Part print with two shaded views. Sizes in mm from the minimum x, y, z corner. Coordinates: 2 decimals unless noted, no trailing zeros. Write each loop counter-clockwise with the first axis right and the second up, starting at its lowest first coordinate (ties: lowest second). Pieces come first, ordered by that corner, then holes. Notation, with made-up numbers: (-32.75, 1) - (2.25, 1) arc R36 ccw to (2.25, 36) - close; hole circle Ø4 at (59.5, 25). An arc over 180 degrees is marked (long way). Answer in a Markdown table with one row per item. Add a question column.
Q1. Band-saw the part on A-A (x = 50). List the corners of the cut face in (y, z), and give its area (3 significant figures).
Q2. Band-saw the part on B-B (z = 61). List the corners of the cut face in (x, y), and give its area (3 significant figures).
Q3. Band-saw the part on C-C (y = 0.6). State how many separate pieces and enclosed holes the cut face has, and give its area (3 significant figures).
Q4. Drill centre lines: line 1 along Z through (x, y) = (53, 0.5); line 2 along X through (y, z) = (0.5, 44); line 3 along X through (y, z) = (0.85, 57) (3 decimals). Where is each one in solid material? Low to high. Write a range as from..to.
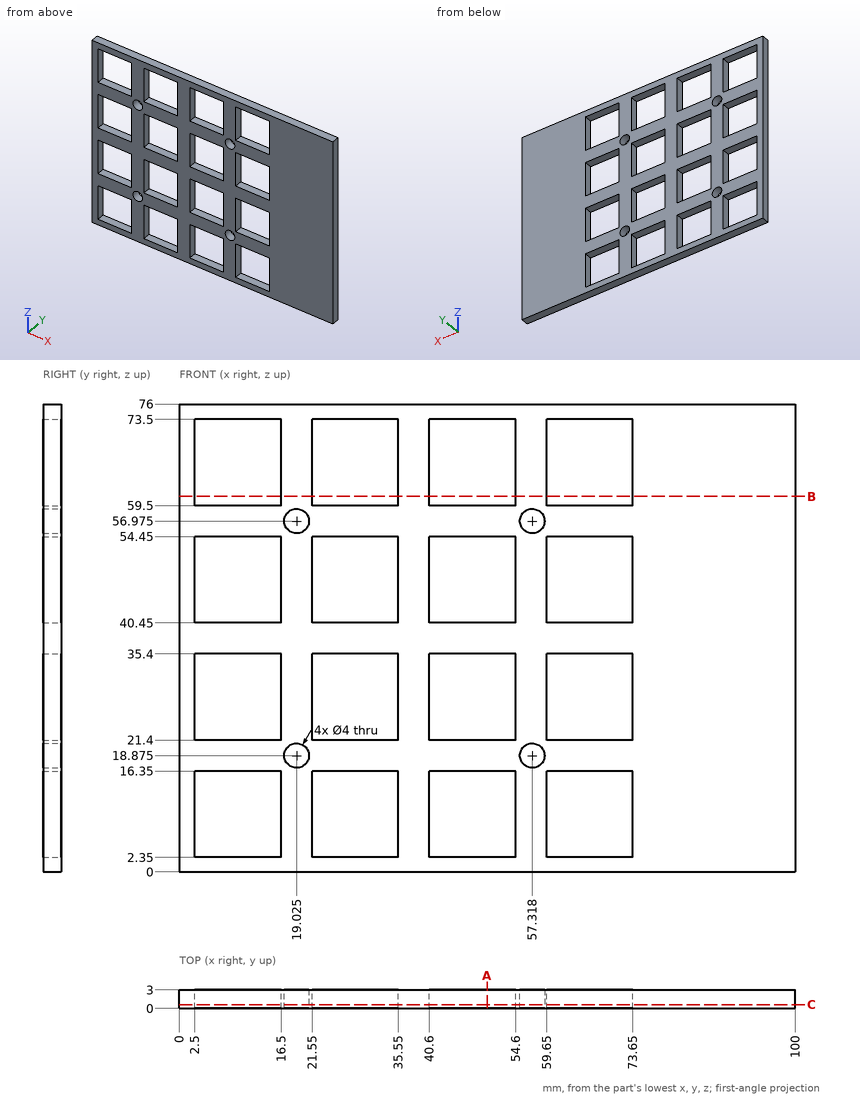
Checked values:
| question | item | result |
|---|---|---|
| 1 | outline | (0, 0) - (3, 0) - (3, 2.35) - (0, 2.35) - close; (0, 16.35) - (3, 16.35) - (3, 21.4) - (0, 21.4) - close; (0, 35.4) - (3, 35.4) - (3, 40.45) - (0, 40.45) - close; (0, 54.45) - (3, 54.45) - (3, 59.5) - (0, 59.5) - close; (0, 73.5) - (3, 73.5) - (3, 76) - (0, 76) - close |
| 1 | area | 60.0 mm² |
| 2 | outline | (0, 0) - (2.5, 0) - (2.5, 3) - (0, 3) - close; (16.5, 0) - (21.55, 0) - (21.55, 3) - (16.5, 3) - close; (35.55, 0) - (40.6, 0) - (40.6, 3) - (35.55, 3) - close; (54.6, 0) - (59.65, 0) - (59.65, 3) - (54.6, 3) - close; (73.65, 0) - (100, 0) - (100, 3) - (73.65, 3) - close |
| 2 | area | 132 mm² |
| 3 | separate pieces | 1 |
| 3 | enclosed holes | 20 |
| 3 | area | 4,410 mm² |
| 4 | line 1 | z = 0..2.35, 16.35..21.4, 35.4..40.45, 54.45..59.5, 73.5..76 |
| 4 | line 2 | x = 0..2.5, 16.5..21.55, 35.55..40.6, 54.6..59.65, 73.65..100 |
| 4 | line 3 | x = 0..17.025, 21.025..55.318, 59.318..100 |
